```python
from build123d import *

# Parameters (mm, degrees)
S_BOX1_W        = 30.8
S_BOX1_H        = 34.5
BOSS_1_DEPTH    = 2.5
S_BOX2_W        = 30.8
S_BOX2_H        = 34.5
BOSS_2_DEPTH    = 2.5
S_BOX3_W        = 2.5
S_BOX3_H        = 34.5
BOSS_3_DEPTH    = 51.4
S_BOX4_W        = 2.5
S_BOX4_H        = 34.5
BOSS_4_DEPTH    = 51.4
S_BOX5_W        = 30.8
S_BOX5_H        = 3
BOSS_5_DEPTH    = 51.4
S_BOX6_W        = 2.5
S_BOX6_H        = 34.5
BOSS_6_DEPTH    = 30.8
S_BOX7_W        = 2.5
S_BOX7_H        = 34.5
BOSS_7_DEPTH    = 30.8
S_BOX8_W        = 51.4
S_BOX8_H        = 34.5
BOSS_8_DEPTH    = 2.5
S_BOX9_W        = 51.4
S_BOX9_H        = 34.5
BOSS_9_DEPTH    = 2.5
S_BOX10_W       = 51.4
S_BOX10_H       = 3
BOSS_10_DEPTH   = 30.8
BOSS_11_DEPTH   = 34.5
S_HOLE12_R      = 10.5
HOLE_12_DEPTH   = 3.2
S_CUT13_W       = 19.4
S_CUT13_H       = 3.15
POCKET_13_DEPTH = 19.5
S_CUT14_W       = 16.4
S_CUT14_H       = 3.15
POCKET_14_DEPTH = 8.3
S_CUT15_W       = 7
S_CUT15_H       = 3.15
POCKET_15_DEPTH = 11
S_HOLE16_R      = 1.1
HOLE_16_DEPTH   = 3.2
S_HOLE17_R      = 1.1
HOLE_17_DEPTH   = 3.2
S_HOLE18_R      = 1.1
HOLE_18_DEPTH   = 3.2
S_HOLE19_R      = 1.1
HOLE_19_DEPTH   = 3.2
S_HOLE20_R      = 10.5
HOLE_20_DEPTH   = 3.2
S_CUT21_W       = 19.5
S_CUT21_H       = 3.15
POCKET_21_DEPTH = 19.4
S_CUT22_W       = 8.3
S_CUT22_H       = 3.15
POCKET_22_DEPTH = 16.4
S_CUT23_W       = 11
S_CUT23_H       = 3.15
POCKET_23_DEPTH = 7
S_HOLE24_R      = 1.1
HOLE_24_DEPTH   = 3.2
S_HOLE25_R      = 1.1
HOLE_25_DEPTH   = 3.2
S_HOLE26_R      = 1.1
HOLE_26_DEPTH   = 3.2
S_HOLE27_R      = 1.1
HOLE_27_DEPTH   = 3.2


with BuildPart() as part:
    # S_box1 → Boss_1 (new body)
    with BuildSketch(Plane.XY.offset(-38.2)):
        with Locations((0, 20.15)):
            Rectangle(S_BOX1_W, S_BOX1_H)
    extrude(amount=BOSS_1_DEPTH)



with BuildPart() as body_2:
    # S_box2 → Boss_2 (new body)
    with BuildSketch(Plane.XY.offset(10.7)):
        with Locations((0, 20.15)):
            Rectangle(S_BOX2_W, S_BOX2_H)
    extrude(amount=BOSS_2_DEPTH)


with BuildPart() as part_1:
    add(part.part)

    add(body_2.part)  # Boss_3 merges body 2
    # S_box3 → Boss_3 (add)
    with BuildSketch(Plane.XY.offset(-38.2)):
        with Locations((-14.15, 20.15)):
            Rectangle(S_BOX3_W, S_BOX3_H)
    extrude(amount=BOSS_3_DEPTH)

    # S_box4 → Boss_4 (add)
    with BuildSketch(Plane.XY.offset(-38.2)):
        with Locations((14.15, 20.15)):
            Rectangle(S_BOX4_W, S_BOX4_H)
    extrude(amount=BOSS_4_DEPTH)

    # S_box5 → Boss_5 (add)
    with BuildSketch(Plane.XY.offset(-38.2)):
        with Locations((0, 35.9)):
            Rectangle(S_BOX5_W, S_BOX5_H)
    extrude(amount=BOSS_5_DEPTH)

    # S_box6 → Boss_6 (add)
    with BuildSketch(Plane.XY.offset(-67.4)):
        with Locations((-11.95, 20.85)):
            Rectangle(S_BOX6_W, S_BOX6_H)
    extrude(amount=BOSS_6_DEPTH)



with BuildPart() as body_2_2:
    # S_box7 → Boss_7 (new body)
    with BuildSketch(Plane.XY.offset(-67.4)):
        with Locations((36.95, 20.85)):
            Rectangle(S_BOX7_W, S_BOX7_H)
    extrude(amount=BOSS_7_DEPTH)


with BuildPart() as part_2:
    add(part_1.part)

    add(body_2_2.part)  # Boss_8 merges body 2 2
    # S_box8 → Boss_8 (add)
    with BuildSketch(Plane.XY.offset(-67.4)):
        with Locations((12.5, 20.85)):
            Rectangle(S_BOX8_W, S_BOX8_H)
    extrude(amount=BOSS_8_DEPTH)

    # S_box9 → Boss_9 (add)
    with BuildSketch(Plane.XY.offset(-39.1)):
        with Locations((12.5, 20.85)):
            Rectangle(S_BOX9_W, S_BOX9_H)
    extrude(amount=BOSS_9_DEPTH)

    # S_box10 → Boss_10 (add)
    with BuildSketch(Plane.XY.offset(-67.4)):
        with Locations((12.5, 5.1)):
            Rectangle(S_BOX10_W, S_BOX10_H)
    extrude(amount=BOSS_10_DEPTH)

    # S_prism11 → Boss_11 (add)
    with BuildSketch(Plane(origin=(0, 2.9, 0), x_dir=(1, 0, 0), z_dir=(0, 1, 0))):
        with BuildLine():
            Line((-15.45, -10.75), (15.45, -10.75))
            Line((15.45, -10.75), (15.45, -11.2))
            ThreePointArc((15.45, -11.2), (13.6926, -15.4426), (9.45, -17.2))
            Line((9.45, -17.2), (-9.45, -17.2))
            ThreePointArc((-9.45, -17.2), (-13.6926, -15.4426), (-15.45, -11.2))
            Line((-15.45, -11.2), (-15.45, -10.75))
        make_face()
    extrude(amount=BOSS_11_DEPTH)

    # S_hole12 → Hole_12 (cut)
    with BuildSketch(Plane(origin=(0, 34.3, 0), x_dir=(1, 0, 0), z_dir=(0, 1, 0))):
        with Locations(Location((0, 0, 0), (0, 0, 90))):
            Circle(S_HOLE12_R)
    extrude(amount=HOLE_12_DEPTH, mode=Mode.SUBTRACT)

    # S_cut13 → Pocket_13 (cut)
    with BuildSketch(Plane.XY.offset(-30.4)):
        with Locations((0, 35.925)):
            Rectangle(S_CUT13_W, S_CUT13_H)
    extrude(amount=POCKET_13_DEPTH, mode=Mode.SUBTRACT)

    # S_cut14 → Pocket_14 (cut)
    with BuildSketch(Plane.XY.offset(-38.7)):
        with Locations((0, 35.925)):
            Rectangle(S_CUT14_W, S_CUT14_H)
    extrude(amount=POCKET_14_DEPTH, mode=Mode.SUBTRACT)

    # S_cut15 → Pocket_15 (cut)
    with BuildSketch(Plane.XY.offset(-11)):
        with Locations((0, 35.925)):
            Rectangle(S_CUT15_W, S_CUT15_H)
    extrude(amount=POCKET_15_DEPTH, mode=Mode.SUBTRACT)

    # S_hole16 → Hole_16 (cut)
    with BuildSketch(Plane(origin=(0, 34.3, 0), x_dir=(1, 0, 0), z_dir=(0, 1, 0))):
        with Locations(Location((-10.25, 8.3, 0), (0, 0, 90))):
            Circle(S_HOLE16_R)
    extrude(amount=HOLE_16_DEPTH, mode=Mode.SUBTRACT)

    # S_hole17 → Hole_17 (cut)
    with BuildSketch(Plane(origin=(0, 34.3, 0), x_dir=(1, 0, 0), z_dir=(0, 1, 0))):
        with Locations(Location((10.25, 8.3, 0), (0, 0, 90))):
            Circle(S_HOLE17_R)
    extrude(amount=HOLE_17_DEPTH, mode=Mode.SUBTRACT)

    # S_hole18 → Hole_18 (cut)
    with BuildSketch(Plane(origin=(0, 34.3, 0), x_dir=(1, 0, 0), z_dir=(0, 1, 0))):
        with Locations(Location((-10.25, 32.75, 0), (0, 0, 90))):
            Circle(S_HOLE18_R)
    extrude(amount=HOLE_18_DEPTH, mode=Mode.SUBTRACT)

    # S_hole19 → Hole_19 (cut)
    with BuildSketch(Plane(origin=(0, 34.3, 0), x_dir=(1, 0, 0), z_dir=(0, 1, 0))):
        with Locations(Location((10.25, 32.75, 0), (0, 0, 90))):
            Circle(S_HOLE19_R)
    extrude(amount=HOLE_19_DEPTH, mode=Mode.SUBTRACT)

    # S_hole20 → Hole_20 (cut)
    with BuildSketch(Plane(origin=(0, 3.5, 0), x_dir=(1, 0, 0), z_dir=(0, 1, 0))):
        with Locations(Location((0, 52, 0), (0, 0, 90))):
            Circle(S_HOLE20_R)
    extrude(amount=HOLE_20_DEPTH, mode=Mode.SUBTRACT)

    # S_cut21 → Pocket_21 (cut)
    with BuildSketch(Plane.XY.offset(-61.7)):
        with Locations((20.65, 5.075)):
            Rectangle(S_CUT21_W, S_CUT21_H)
    extrude(amount=POCKET_21_DEPTH, mode=Mode.SUBTRACT)

    # S_cut22 → Pocket_22 (cut)
    with BuildSketch(Plane.XY.offset(-60.2)):
        with Locations((34.55, 5.075)):
            Rectangle(S_CUT22_W, S_CUT22_H)
    extrude(amount=POCKET_22_DEPTH, mode=Mode.SUBTRACT)

    # S_cut23 → Pocket_23 (cut)
    with BuildSketch(Plane.XY.offset(-55.5)):
        with Locations((5.5, 5.075)):
            Rectangle(S_CUT23_W, S_CUT23_H)
    extrude(amount=POCKET_23_DEPTH, mode=Mode.SUBTRACT)

    # S_hole24 → Hole_24 (cut)
    with BuildSketch(Plane(origin=(0, 3.5, 0), x_dir=(1, 0, 0), z_dir=(0, 1, 0))):
        with Locations(Location((8.3, 62.25, 0), (0, 0, 90))):
            Circle(S_HOLE24_R)
    extrude(amount=HOLE_24_DEPTH, mode=Mode.SUBTRACT)

    # S_hole25 → Hole_25 (cut)
    with BuildSketch(Plane(origin=(0, 3.5, 0), x_dir=(1, 0, 0), z_dir=(0, 1, 0))):
        with Locations(Location((8.3, 41.75, 0), (0, 0, 90))):
            Circle(S_HOLE25_R)
    extrude(amount=HOLE_25_DEPTH, mode=Mode.SUBTRACT)

    # S_hole26 → Hole_26 (cut)
    with BuildSketch(Plane(origin=(0, 3.5, 0), x_dir=(1, 0, 0), z_dir=(0, 1, 0))):
        with Locations(Location((32.75, 62.25, 0), (0, 0, 90))):
            Circle(S_HOLE26_R)
    extrude(amount=HOLE_26_DEPTH, mode=Mode.SUBTRACT)

    # S_hole27 → Hole_27 (cut)
    with BuildSketch(Plane(origin=(0, 3.5, 0), x_dir=(1, 0, 0), z_dir=(0, 1, 0))):
        with Locations(Location((32.75, 41.75, 0), (0, 0, 90))):
            Circle(S_HOLE27_R)
    extrude(amount=HOLE_27_DEPTH, mode=Mode.SUBTRACT)


solid = part_2.part
```
The model under review builds one solid part; all positions refer to its coordinate system, in mm. A direction names the side the tool comes from. Coordinates: 2 decimals unless noted, no trailing zeros. Write each loop counter-clockwise with the first axis right and the second up, starting at its lowest first coordinate (ties: lowest second). Pieces come first, ordered by that corner, then holes. Notation, with made-up numbers: (18.5, 60) - (43.5, 60) arc R32 cw to (43.5, 89) - close; hole circle Ø1 at (72.25, 47). An arc over 180 degrees is marked (long way). Write item = value, one per line.
(1) Consider section C-C, the plane z = -21. Give the boundary of the cut face in (x, y), then the cut area to 3 significant figures.
Result sheet:
outline = (-15.4, 2.9) - (-12.9, 2.9) - (-12.9, 34.4) - (-9.7, 34.4) - (-9.7, 37.4) - (-15.4, 37.4) - close; (9.7, 34.4) - (12.9, 34.4) - (12.9, 2.9) - (15.4, 2.9) - (15.4, 37.4) - (9.7, 37.4) - close
area = 192 mm^2
(2) Consider section D-D, the plane y = 32. Give the boundary of the cut face in (x, z).
Result sheet:
outline = (-15.45, 10.75) - (-15.4, 10.75) - (-15.4, -38.2) - (-13.2, -38.2) - (-13.2, -67.4) - (38.2, -67.4) - (38.2, -36.6) - (15.4, -36.6) - (15.4, 10.75) - (15.45, 10.75) - (15.45, 11.2) arc R6 ccw to (15.4, 11.97) - (15.4, 13.2) - (15.11, 13.2) arc R6 ccw to (9.45, 17.2) - (-9.45, 17.2) arc R6 ccw to (-15.11, 13.2) - (-15.4, 13.2) - (-15.4, 11.97) arc R6 ccw to (-15.45, 11.2) - close; hole (-12.9, -35.7) - (12.9, -35.7) - (12.9, 10.7) - (-12.9, 10.7) - close; hole (-10.7, -64.9) - (35.7, -64.9) - (35.7, -39.1) - (-10.7, -39.1) - close
(3) Machinability: for faces 1 (the face through (10.9, 5, -45)), 2 (the face through (8.2, 36, -35)), 3 (the face through (34, 5, -60.2)), 4 (the face through (0, 19, 10.7)), which of the approach directions +Z, -Z, +X, -X, +Y, -Y give a long, thin tool a straight path to every point of the face, cutting with its end or side? Answer none if there is none.
Result sheet:
face_1 = +Y, -Y
face_2 = none
face_3 = +X, -Y
face_4 = -Y
(4) Consider section B-B, the plane x = 32.75. Give the boundary of the cut face in (y, z).
Result sheet:
outline = (3.6, -67.4) - (38.1, -67.4) - (38.1, -64.9) - (6.6, -64.9) - (6.6, -63.35) - (3.6, -63.35) - close; (3.6, -61.15) - (6.6, -61.15) - (6.6, -60.2) - (3.6, -60.2) - close; (3.6, -43.8) - (6.6, -43.8) - (6.6, -42.85) - (3.6, -42.85) - close; (3.6, -40.65) - (6.6, -40.65) - (6.6, -39.1) - (38.1, -39.1) - (38.1, -36.6) - (3.6, -36.6) - close
(5) For P1, Ø3.5, axis at y = 5, z = -59.5, coming from the +X side; P2, Ø3.5, axis at x = 24, y = 5.5, coming from the +Z side; P3, Ø16, axis at y = 21, z = -7, coming from the -X side; P4, Ø8, axis at y = 14, z = -17, coming from the +X side, all flat-tipped, find the tip position at first contact; note any pin that passes through.
Result sheet:
P1 = 38.2
P2 = -36.6
P3 = -15.4
P4 = 15.4
(6) Mouldability with a two-part tool opening along X and no side actions: class faces 5 (the face through (11, 37.4, -11)), 6 (the face through (12, 23, -64.9)), 7 (the face through (38.2, 21, -52)) as pulls with the +X half, pulls with the -X half, needs draft (parallel to the pull), parting line crosses it, or undercut.
Result sheet:
face_5 = needs draft
face_6 = undercut
face_7 = pulls with the +X half
(7) For line 1 (X direction, y = 36.2, z = -32.75); line 2 (Z direction, x = 0, y = 30); line 3 (Z direction, x = 24, y = 8), list the stretches that pass through material, from the lowest coordinate up. Write a range as [from, to].
Result sheet:
line_1 = [-15.4, -11.35], [-9.15, -8.2], [8.2, 9.15], [11.35, 15.4]
line_2 = [-67.4, -64.9], [-39.1, -35.7], [10.7, 17.2]
line_3 = [-67.4, -64.9], [-39.1, -36.6]
(8) Consider section A-A, the plane z = -32.75. Give the boundary of the cut face in (x, y).
Result sheet:
outline = (-15.4, 2.9) - (-12.9, 2.9) - (-12.9, 34.4) - (-11.35, 34.4) - (-11.35, 37.4) - (-15.4, 37.4) - close; (-9.15, 34.4) - (-8.2, 34.4) - (-8.2, 37.4) - (-9.15, 37.4) - close; (8.2, 34.4) - (9.15, 34.4) - (9.15, 37.4) - (8.2, 37.4) - close; (11.35, 34.4) - (12.9, 34.4) - (12.9, 2.9) - (15.4, 2.9) - (15.4, 37.4) - (11.35, 37.4) - close
